The listing builds one solid part. Answer for the finished solid, in the listing's coordinates (mm). A direction names the side the tool comes from. Round coordinates to 2 decimals unless told otherwise and drop trailing zeros. Loops run counter-clockwise (first coordinate to the right, second up) from the corner with the lowest first, then second, coordinate; pieces in that order, holes last. Notation, with made-up numbers: (-27, 30) - (-8, 30) arc R29 cw to (-8, 59) - close; hole circle Ø8 at (64.25, 1). An arc over 180 degrees is marked (long way). One line per item, written item: value.
```python
from build123d import *

# Parameters (mm, degrees)
SKETCH1_R           = 15
BOSS_EXTRUDE1_DEPTH = 1.3
BOSS_EXTRUDE2_START = -1.65
SKETCH1_3_R         = 15
SKETCH1_3_R_2       = 10.75
BOSS_EXTRUDE2_DEPTH = 1.65
CUT_EXTRUDE1_START  = -10
SKETCH1_5_R         = 10.75
SKETCH1_5_R_2       = 6.2
CUT_EXTRUDE1_DEPTH  = 10
FILLET5_R           = 0.5
FILLET6_R           = 0.5


with BuildPart() as part:
    # Sketch1 → Boss-Extrude1 (new body)
    with BuildSketch(Plane(origin=(0, 0, 0), x_dir=(1, 0, 0), z_dir=(0, 1, 0))):
        with Locations(Location((0, 0, 0), (0, 0, 270))):
            Circle(SKETCH1_R)
        with BuildLine():
            ThreePointArc((-13.2, 0), (-9.727636339, 5.567764363), (-3.2, 4.898979486))
            Line((-3.2, 4.898979486), (-3.2, -4.898979486))
            ThreePointArc((-3.2, -4.898979486), (-9.727636339, -5.567764363), (-13.2, 0))
        make_face(mode=Mode.SUBTRACT)
        with BuildLine():
            Line((3.071845277, -4.91349301), (3.034307887, 4.884394056))
            ThreePointArc((3.034307887, 4.884394056), (13.053003194, 0.023761962), (3.071845277, -4.91349301))
        make_face(mode=Mode.SUBTRACT)
    extrude(amount=BOSS_EXTRUDE1_DEPTH)

    # Sketch1<3> → Boss-Extrude2 (add)
    with BuildSketch(Plane(origin=(0, 0, 0), x_dir=(1, 0, 0), z_dir=(0, 1, 0)).offset(BOSS_EXTRUDE2_START)):
        with Locations(Location((0, 0, 0), (0, 0, 270))):
            Circle(SKETCH1_3_R)
        with Locations(Location((0, 0, 0), (0, 0, 270))):
            Circle(SKETCH1_3_R_2, mode=Mode.SUBTRACT)
    extrude(amount=BOSS_EXTRUDE2_DEPTH)

    # Sketch1<5> → Cut-Extrude1 (cut)
    with BuildSketch(Plane(origin=(0, 0, 0), x_dir=(1, 0, 0), z_dir=(0, 1, 0)).offset(CUT_EXTRUDE1_START)):
        with BuildLine():
            ThreePointArc((-9.00875, -5.865571024), (-10.305497623, -3.059284026), (-10.75, 0))
            Line((-10.75, 0), (-13.2, 0))
            ThreePointArc((-13.2, 0), (-12.044514347, -3.60456308), (-9.00875, -5.865571024))
        make_face()
        with BuildLine():
            Line((-13.2, 0), (-10.75, 0))
            ThreePointArc((-10.75, 0), (-10.305497623, 3.059284026), (-9.00875, 5.865571024))
            ThreePointArc((-9.00875, 5.865571024), (-12.044514347, 3.60456308), (-13.2, 0))
        make_face()
        Circle(SKETCH1_5_R)
        with Locations((6.853048695, 8.87e-06)):
            Circle(SKETCH1_5_R_2)
    extrude(amount=CUT_EXTRUDE1_DEPTH, mode=Mode.SUBTRACT)

    # Fillet5
    fillet5_edges = [part.edges().sort_by_distance(p)[0] for p in [
        (-3.2, 1.3, 0),
        (13.053003194, 1.3, -0.023761962),
        (3.053076582, 1.3, 0.014549477),
        (-13.2, 1.3, 0),
    ]]
    fillet(fillet5_edges, radius=FILLET5_R)

    # Fillet6
    fillet6_edges = [part.edges().sort_by_distance(p)[0] for p in [
        (0, -1.65, -15),
        (0.041164562, -1.65, 10.749921185),
    ]]
    fillet(fillet6_edges, radius=FILLET6_R)


solid = part.part
```
1) Each of these flat-tipped pins is pushed along its axis until it touches: pin 1 Ø5 at (x, z) = (-6, -1) entering from +Y; pin 2 Ø1.5 at (x, y) = (-6.5, 0) entering from -Z; pin 3 Ø1.5 at (x, y) = (1, 0) entering from +Z; pin 4 Ø0.6 at (y, z) = (0.5, 2.5) entering from -X. Where does it stop, or does it pass through?
Final values:
pin 1: through
pin 2: z = -13.85
pin 3: z = 15
pin 4: x = -14.84
2) For a pull along Z with two mould halves and no side action, classify faces 4 (the cylindrical face through (0.66, 0.058, -14.985)), 5 (the cylindrical face through (0.19, -0.84, -10.75)), 6 (the cylindrical face through (-0.11, -0.58, 10.75)), 7 (the flat face through (9, -1.65, -7)) as released by +Z, released by -Z, zero draft, split by the parting line, or undercut.
Final values:
face 4: split by the parting line
face 5: undercut
face 6: undercut
face 7: zero draft
3) For faces 1 (the flat face through (0, 1.3, 0)), 2 (the flat face through (-3.2, 0.4, -0.1)), 3 (the flat face through (0, 0, 0)), determine the directions among +Z, -Z, +X, -X, +Y, -Y from which every point of the face is accessible in a straight line to the end or side of a thin tool.
Final values:
face 1: +Z, -Z, +X, -X, +Y
face 2: +Y, -Y
face 3: -Y
4) Consider L1, parallel to X at y = 1, z = 3; L2, parallel to X at y = 0.35, z = 2; L3, parallel to X at y = -0.85, z = 8. Determine where each line is inside the solid, lowest interval first.
Final values:
L1: -14.7 to -12.47, -3.16 to 3.02, 12.33 to 14.7
L2: -14.87 to -12.87, -3.2 to 3.06, 12.72 to 14.87
L3: -12.69 to -7.18, 7.18 to 12.69
5) A cutting plane is placed at A-A on x = 0. Give the vertices of the cut face in (y, z), and give its area (3 significant figures).
Final values:
outline: (-1.65, -14.5) arc R0.5 ccw to (-1.15, -15) - (1.3, -15) - (1.3, 15) - (-1.15, 15) arc R0.5 ccw to (-1.65, 14.5) - (-1.65, 11.25) arc R0.5 ccw to (-1.15, 10.75) - (0, 10.75) - (0, -10.75) - (-1.65, -10.75) - close
area: 52.9 mm2
6) A cutting plane is placed at B-B on z = 1. Give the number of separate pieces and of enclosed holes in the cut face, and give its area (3 significant figures).
Final values:
separate pieces: 3
enclosed holes: 0
area: 19.1 mm2
